Geometry check sheet. Reference: the model listing, model coordinates, mm. A direction names the side the tool comes from. Give positions to 0.01 mm unless a question says otherwise; leave off trailing zeros. Loops run counter-clockwise (first coordinate to the right, second up) from the corner with the lowest first, then second, coordinate; pieces in that order, holes last.
```python
from build123d import *

# Parameters (mm, degrees)
SKETCH1_W           = 125
SKETCH1_H           = 125
SKETCH1_W_2         = 120
SKETCH1_H_2         = 120
BOSS_EXTRUDE1_DEPTH = 100
SKETCH3_W           = 10
SKETCH3_H           = 10
BOSS_EXTRUDE2_DEPTH = 70
SKETCH4_R           = 2.5
CUT_EXTRUDE1_DEPTH  = 5
SKETCH5_W           = 120
SKETCH5_H           = 120
CUT_EXTRUDE2_DEPTH  = 65


with BuildPart() as part:
    # Sketch1 → Boss-Extrude1 (new body)
    with BuildSketch(Plane(origin=(0, 0, 0), x_dir=(1, 0, 0), z_dir=(0, 1, 0))):
        Rectangle(SKETCH1_W, SKETCH1_H)
        Rectangle(SKETCH1_W_2, SKETCH1_H_2, mode=Mode.SUBTRACT)
    extrude(amount=BOSS_EXTRUDE1_DEPTH)

    # Sketch3 → Boss-Extrude2 (add)
    with BuildSketch(Plane(origin=(0, 100, 0), x_dir=(1, 0, 0), z_dir=(0, 1, 0))):
        with Locations((55, 55)):
            Rectangle(SKETCH3_W, SKETCH3_H)
        with Locations((-55, 55)):
            Rectangle(SKETCH3_W, SKETCH3_H)
        with Locations((55, -55)):
            Rectangle(SKETCH3_W, SKETCH3_H)
        with Locations((-55, -55)):
            Rectangle(SKETCH3_W, SKETCH3_H)
    extrude(amount=-BOSS_EXTRUDE2_DEPTH)

    # Sketch4 → Cut-Extrude1 (cut)
    with BuildSketch(Plane.XZ.offset(-30)):
        with Locations((-55, 55)):
            Circle(SKETCH4_R)
        with Locations((55, 55)):
            Circle(SKETCH4_R)
        with Locations((55, -55)):
            Circle(SKETCH4_R)
        with Locations((-55, -55)):
            Circle(SKETCH4_R)
    extrude(amount=-CUT_EXTRUDE1_DEPTH, mode=Mode.SUBTRACT)

    # Sketch5 → Cut-Extrude2 (cut)
    with BuildSketch(Plane(origin=(0, 100, 0), x_dir=(1, 0, 0), z_dir=(0, 1, 0))):
        Rectangle(SKETCH5_W, SKETCH5_H)
    extrude(amount=-CUT_EXTRUDE2_DEPTH, mode=Mode.SUBTRACT)


solid = part.part
```
1) Mould release check, pull along Z, two halves, no side actions. Record for faces 6 (the flat face through (-1, 49, -62.5)), 7 (the flat face through (-60.5, 0, -28.1)), 8 (the flat face through (-55, 33, 50)): +Z half, -Z half, draft (parallel to the pull), parting line (faces both ways), or undercut.
2) Depth check by flat-ended pin: P1, Ø5, axis at x = -53, z = 54, coming from the +Y side. Enter the tip coordinate at first touch or a pass-through.
3) Sectioned sample at A-A on z = -55. Enter the section's corners in (x, y), plus the area to 3 significant figures.
4) Scan lines: line 1 along Z through (x, y) = (55, 32); line 2 along Z through (x, y) = (-30, 26). Record each from-to range of solid material in increasing order.
5) Tool access check on faces 1 (the flat face through (-55, 33, -50)), 2 (the flat face through (-62.5, 49, 1)), 3 (the flat face through (-57, 30, 53)), 4 (the flat face through (-1, 49, 62.5)), 5 (the flat face through (-57, 35, 53)). Record the directions out of +Z, -Z, +X, -X, +Y, -Y that give a thin tool (end or side, any length) a straight path to the whole face; none if there is none.
6) Sectioned sample at D-D on z = 32. Enter the section's corners in (x, y), plus the area to 3 significant figures.
7) Sectioned sample at C-C on y = 32.5. Enter the section's corners in (x, z).
8) Sectioned sample at B-B on x = -41.5. Enter the section's corners in (y, z), plus the area to 3 significant figures.
Determined:
1. face 6: -Z half
1. face 7: draft
1. face 8: undercut
2. P1: stops at y = 35
3. outline: (-62.5, 0) - (-60, 0) - (-60, 30) - (-57.5, 30) - (-57.5, 35) - (-60, 35) - (-60, 100) - (-62.5, 100) - close; (-52.5, 30) - (-50, 30) - (-50, 35) - (-52.5, 35) - close; (50, 30) - (52.5, 30) - (52.5, 35) - (50, 35) - close; (57.5, 30) - (60, 30) - (60, 0) - (62.5, 0) - (62.5, 100) - (60, 100) - (60, 35) - (57.5, 35) - close
3. area: 550 mm2
4. line 1: z = -62.5 to -57.5, -52.5 to -50, 50 to 52.5, 57.5 to 62.5
4. line 2: z = -62.5 to -60, 60 to 62.5
5. face 1: +Y, -Y
5. face 2: +Z, -Z, -X, +Y, -Y
5. face 3: -Y
5. face 4: +Z, +X, -X, +Y, -Y
5. face 5: +Y
6. outline: (-62.5, 0) - (-60, 0) - (-60, 100) - (-62.5, 100) - close; (60, 0) - (62.5, 0) - (62.5, 100) - (60, 100) - close
6. area: 500 mm2
7. outline: (-62.5, -62.5) - (62.5, -62.5) - (62.5, 62.5) - (-62.5, 62.5) - close; hole (-60, -50) - (-50, -50) - (-50, -60) - (50, -60) - (50, -50) - (60, -50) - (60, 50) - (50, 50) - (50, 60) - (-50, 60) - (-50, 50) - (-60, 50) - close; hole circle Ø5 at (-55, -55); hole circle Ø5 at (-55, 55); hole circle Ø5 at (55, -55); hole circle Ø5 at (55, 55)
8. outline: (0, -62.5) - (100, -62.5) - (100, -60) - (0, -60) - close; (0, 60) - (100, 60) - (100, 62.5) - (0, 62.5) - close
8. area: 500 mm2
